```python
from build123d import *

# Parameters (mm, degrees)
F0_W     = 40.64
F0_H     = 76.2
F1_DEPTH = 50.8
F2_R     = 31.75
F3_R     = 31.75
F4_R     = 25.4


with BuildPart() as f1:
    # F0 (on Top) → F1 (new body)
    with BuildSketch(Plane.XY):
        Polygon((0, 76.2), (0, 0), (40.64, 0), (111.76, 0), (152.4, 0), (152.4, 76.2), align=None)
        with Locations((20.32, -38.1)):
            Rectangle(F0_W, F0_H)
        with Locations((132.08, -38.1)):
            Rectangle(F0_W, F0_H)
    extrude(amount=F1_DEPTH)

    # F2
    f2_edges = [f1.edges().sort_by_distance(p)[0] for p in [
        (20.32, -76.2, 50.8),
        (132.08, -76.2, 50.8),
    ]]
    fillet(f2_edges, radius=F2_R)

    # F3
    f3_edges = [f1.edges().sort_by_distance(p)[0] for p in [
        (152.4, 76.2, 25.4),
        (0, 76.2, 25.4),
    ]]
    fillet(f3_edges, radius=F3_R)

    # F4
    f4_edges = [f1.edges().sort_by_distance(p)[0] for p in [
        (111.76, 0, 25.4),
        (40.64, 0, 25.4),
    ]]
    fillet(f4_edges, radius=F4_R)


solid = f1.part
```
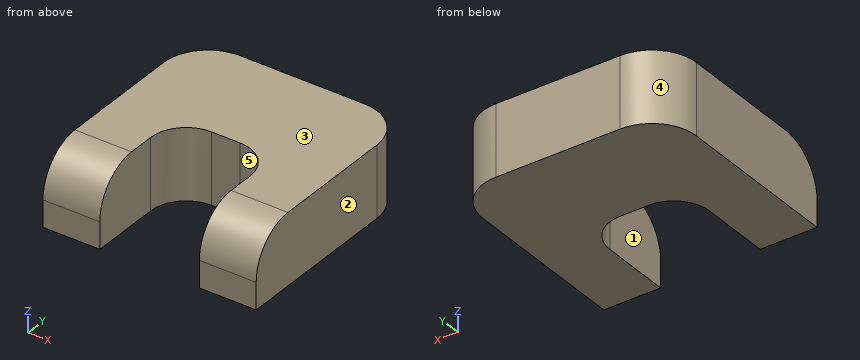
Check sheet for the modelled part. Datum: model origin and axes. Units: mm. Face numbers are marked on the shaded views. A direction names the side the tool comes from. Coordinates: 2 decimals unless noted, no trailing zeros. Order: outer loops, then holes, each group sorted by start corner. A loop starts at its lowest first (then second) coordinate and runs counter-clockwise, first axis right, second up. Notation, with made-up numbers: (30, 12) -> (83, 12) arc R27 cw to (83, 45) -> close; hole circle Ø6 at (71, 42). An arc over 180 degrees is marked (long way). Write item = value, one per line. Start each with the question number.
1) Cross-section at A-A (z = 34). Enter the section's corners in (x, y).
2) Cross-section at D-D (z = 15.5). Enter the section's corners in (x, y), then the cut area to 3 significant figures.
3) Cross-section at C-C (x = 114.5). Enter the section's corners in (y, z), then the cut area to 3 significant figures.
4) Material ranges on L1, parallel to X at y = -59, z = 26.5; L2, parallel to X at y = -15.5, z = 43; L3, parallel to Y at x = 85, z = 8, recorded low to high.
5) Cross-section at B-B (y = -60). Enter the section's corners in (x, z), then the cut area to 3 significant figures.
6) Mould release check, pull along X, two halves, no side actions. Record for the marked faces 1, 2 and 3: +X half, -X half, draft (parallel to the pull), parting line (faces both ways), or undercut.
7) Go/stop test with flat-tipped pins: P1, Ø22.5, axis at x = 79, z = 38, coming from the -Y side; P2, Ø4, axis at x = 124, z = 29.5, coming from the -Y side; P3, Ø1.5, axis at x = 132.5, z = 35.5, coming from the +Y side. Record where each tip stops, or that it passes through.
8) Access from +Z, -Z, +X, -X, +Y, -Y to the whole of each face (thin tool, end or side, straight path). Record for the marked faces 4 and 5.
Ans:
q1.outline = (0, -72.46) -> (40.64, -72.46) -> (40.64, -25.4) arc R25.4 cw to (66.04, 0) -> (86.36, 0) arc R25.4 cw to (111.76, -25.4) -> (111.76, -72.46) -> (152.4, -72.46) -> (152.4, 44.45) arc R31.75 ccw to (120.65, 76.2) -> (31.75, 76.2) arc R31.75 ccw to (0, 44.45) -> close
q2.outline = (0, -76.2) -> (40.64, -76.2) -> (40.64, -25.4) arc R25.4 cw to (66.04, 0) -> (86.36, 0) arc R25.4 cw to (111.76, -25.4) -> (111.76, -76.2) -> (152.4, -76.2) -> (152.4, 44.45) arc R31.75 ccw to (120.65, 76.2) -> (31.75, 76.2) arc R31.75 ccw to (0, 44.45) -> close
q2.area = 17,700 mm²
q3.outline = (-76.2, 0) -> (76.2, 0) -> (76.2, 50.8) -> (-44.45, 50.8) arc R31.75 ccw to (-76.2, 19.05) -> close
q3.area = 7,530 mm²
q4.L1 = 0 to 40.64, 111.76 to 152.4
q4.L2 = 0 to 42.65, 109.75 to 152.4
q4.L3 = 0 to 76.2
q5.outline = (0, 0) -> (40.64, 0) -> (40.64, 46.73) -> (0, 46.73) -> close; (111.76, 0) -> (152.4, 0) -> (152.4, 46.73) -> (111.76, 46.73) -> close
q5.area = 3,800 mm²
q6.face_1 = undercut
q6.face_2 = +X half
q6.face_3 = draft
q7.P1 = -0.3
q7.P2 = -75.05
q7.P3 = 74.2
q8.face_4 = +Z, -Z, -X, +Y
q8.face_5 = +Z, -Z, -Y
